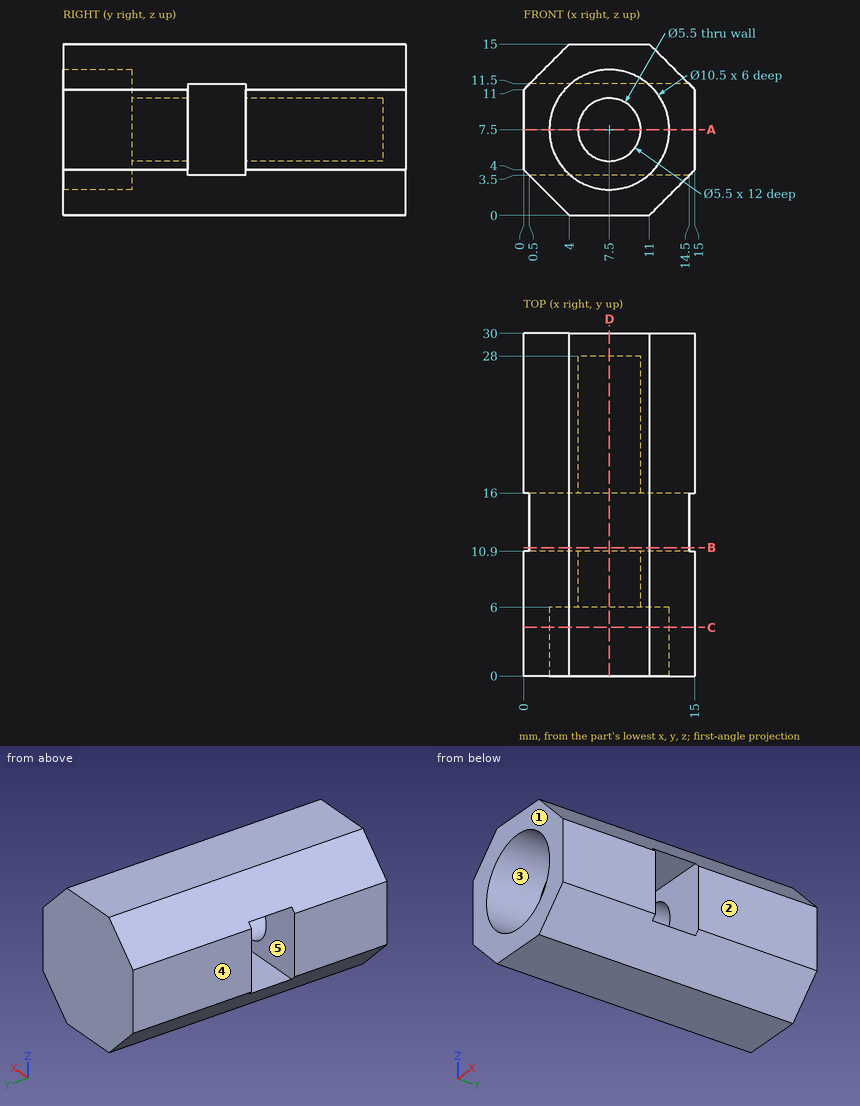
Input: dimensioned drawing with shaded views. Units: mm. Origin: part minimum x, y, z. A direction names the side the tool comes from. Round coordinates to 2 decimals unless told otherwise and drop trailing zeros. Loops run counter-clockwise (first coordinate to the right, second up) from the corner with the lowest first, then second, coordinate; pieces in that order, holes last. Notation, with made-up numbers: (39.25, -21) -> (50.25, -21) arc R11 cw to (50.25, -12) -> close; hole circle Ø11 at (-14, -15.75). An arc over 180 degrees is marked (long way). Answer as a JSON object with one key per item and string values. Group by question number.
1) Reachability of the marked faces 4 and 5 from +Z, -Z, +X, -X, +Y, -Y: full face, straight path, thin tool, end or side. Return the list, or none.
2) Section query B-B on y = 11.25. Output: boundary loops of the cut face in (x, z), plus the area to 3 significant figures.
3) Section query A-A on z = 7.5. Output: boundary loops of the cut face in (x, y), plus the area to 3 significant figures.
4) Ray query, L1, parallel to Z at x = 7.5, y = 7.5; L2, parallel to Z at x = 7.5, y = 3.95; L3, parallel to Y at x = 12.5, z = 6.5. Return the intervals inside material, ascending.
5) Section query C-C on y = 4.25. Output: boundary loops of the cut face in (x, z), plus the area to 3 significant figures.
6) Section query D-D on x = 7.5. Output: boundary loops of the cut face in (y, z), plus the area to 3 significant figures.
7) Pin query (flat end, axial travel): pin 1 (6.5 mm diameter, centred on x = 7.5, z = 7.5, fed in from -Y); pin 2 (4 mm diameter, centred on y = 18.5, z = 13.5, fed in from -X). Return the tip coordinate at first contact, or that it passes through.
8) Draft query along X for the marked faces 1, 2 and 3. Return one class per face: +X half, -X half, draft (parallel to the pull), parting line (faces both ways), or undercut.
Reply:
{
 "1": {"face 4": "+Z, -Z, -X, +Y, -Y", "face 5": "+X, -X"},
 "2": {"outline": "(0.5, 3.5) -> (4, 0) -> (11, 0) -> (14.5, 3.5) -> close; (0.5, 11.5) -> (14.5, 11.5) -> (11, 15) -> (4, 15) -> close", "area": "73.5 mm2"},
 "3": {"outline": "(0, 0) -> (2.25, 0) -> (2.25, 6) -> (4.75, 6) -> (4.75, 10.9) -> (0, 10.9) -> close; (0, 16) -> (4.75, 16) -> (4.75, 28) -> (10.25, 28) -> (10.25, 16) -> (15, 16) -> (15, 30) -> (0, 30) -> close; (10.25, 6) -> (12.75, 6) -> (12.75, 0) -> (15, 0) -> (15, 10.9) -> (10.25, 10.9) -> close", "area": "218 mm2"},
 "4": {"L1": "z = 0 to 4.75, 10.25 to 15", "L2": "z = 0 to 2.25, 12.75 to 15", "L3": "y = 6 to 10.9, 16 to 30"},
 "5": {"outline": "(0, 4) -> (4, 0) -> (11, 0) -> (15, 4) -> (15, 11) -> (11, 15) -> (4, 15) -> (0, 11) -> close; hole circle Ø10.5 at (7.5, 7.5)", "area": "106 mm2"},
 "6": {"outline": "(0, 0) -> (30, 0) -> (30, 15) -> (0, 15) -> (0, 12.75) -> (6, 12.75) -> (6, 10.25) -> (10.9, 10.25) -> (10.9, 11.5) -> (16, 11.5) -> (16, 10.25) -> (28, 10.25) -> (28, 4.75) -> (16, 4.75) -> (16, 3.5) -> (10.9, 3.5) -> (10.9, 4.75) -> (6, 4.75) -> (6, 2.25) -> (0, 2.25) -> close", "area": "253 mm2"},
 "7": {"pin 1": "stops at y = 6", "pin 2": "stops at x = 0.5"},
 "8": {"face 1": "draft", "face 2": "+X half", "face 3": "undercut"}
}
